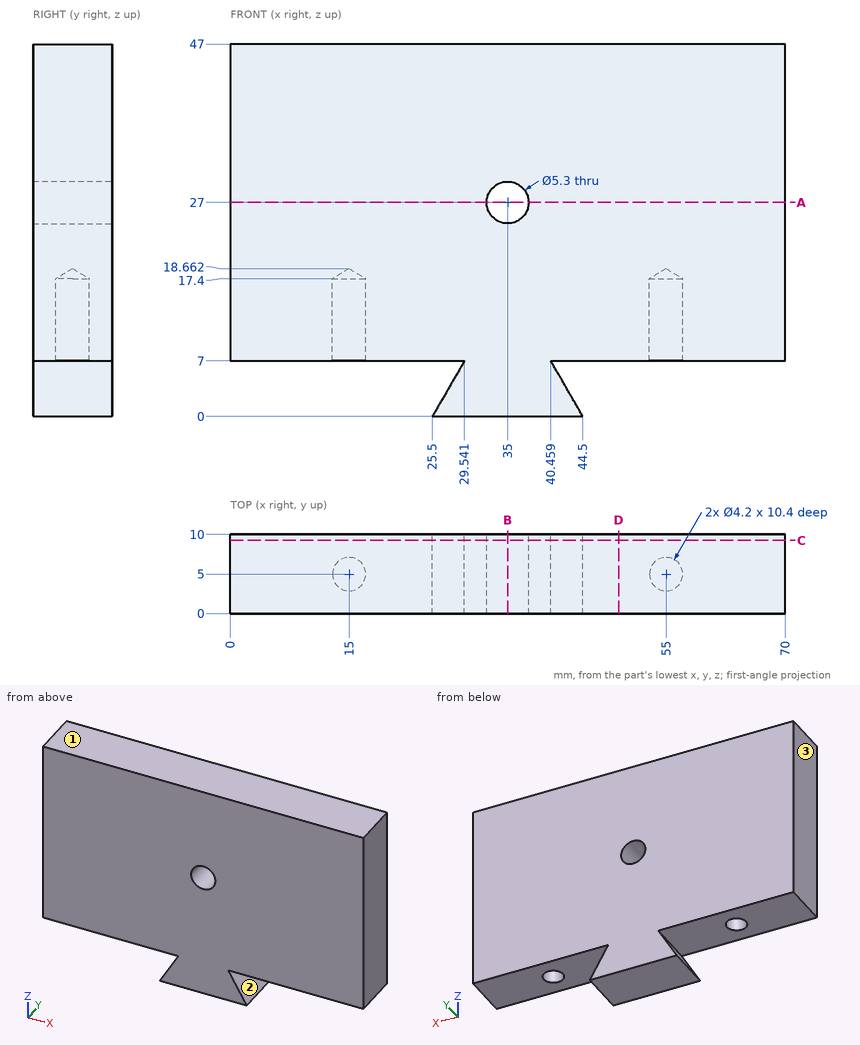
Answer from the drawing. Dimensions are ordinates in mm from the lowest x, y and z of the part. Give positions to 0.01 mm unless a question says otherwise; leave off trailing zeros. Write each loop counter-clockwise with the first axis right and the second up, starting at its lowest first coordinate (ties: lowest second). Pieces come first, ordered by that corner, then holes.
1) Given P1, Ø3, axis at x = 11, y = 5, coming from the -Z side; P2, Ø2, axis at x = 59, z = 5, coming from the +Y side, each flat-ended and moving along its own axis, determine where each tip first touches the part or whether it passes through.
2) Find the intervals of material crossed by L1, parallel to Y at x = 55, z = 11.5; L2, parallel to Z at x = 21, y = 7.5; L3, parallel to X at y = 5.75, z = 8.5, in increasing order.
3) For a pull along Z with two mould halves and no side action, classify the marked faces 1, 2 and 3 as pulls with the +Z half, pulls with the -Z half, needs draft (parallel to the pull), parting line crosses it, or undercut.
4) Section A-A (z = 27) is taken. Write down the section's boundary in (x, y), and give its area (3 significant figures).
5) Section B-B (x = 35) is taken. Write down the section's boundary in (y, z).
6) Section D-D (x = 49) is taken. Write down the section's boundary in (y, z), and give its area (3 significant figures).
7) Section C-C (y = 9.25) is taken. Write down the section's boundary in (x, z).
Response:
1. P1: stops at z = 7
1. P2: passes through
2. L1: y = 0 to 2.9, 7.1 to 10
2. L2: z = 7 to 47
2. L3: x = 0 to 13.04, 16.96 to 53.04, 56.96 to 70
3. face 1: pulls with the +Z half
3. face 2: undercut
3. face 3: needs draft
4. outline: (0, 0) - (32.35, 0) - (32.35, 10) - (0, 10) - close; (37.65, 0) - (70, 0) - (70, 10) - (37.65, 10) - close
4. area: 647 mm2
5. outline: (0, 0) - (10, 0) - (10, 24.35) - (0, 24.35) - close; (0, 29.65) - (10, 29.65) - (10, 47) - (0, 47) - close
6. outline: (0, 7) - (10, 7) - (10, 47) - (0, 47) - close
6. area: 400 mm2
7. outline: (0, 7) - (29.54, 7) - (25.5, 0) - (44.5, 0) - (40.46, 7) - (70, 7) - (70, 47) - (0, 47) - close; hole circle Ø5.3 at (35, 27)
